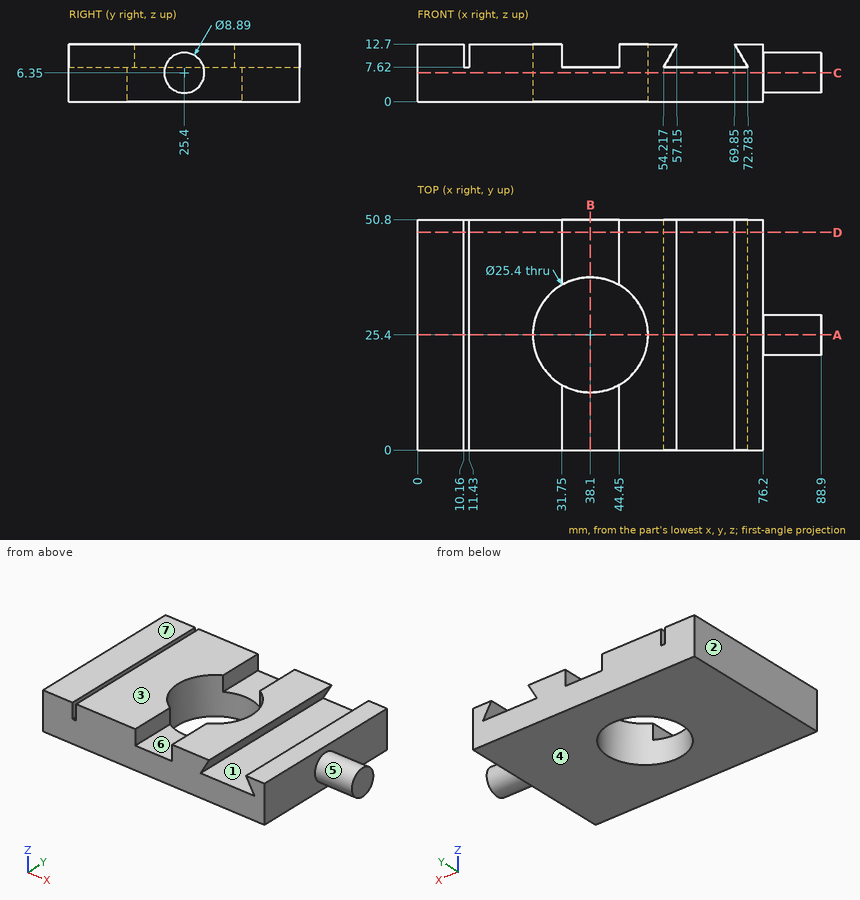
For this review, use the dimensioned drawing (mm, ordinates from the lowest corner) and the shaded views. A direction names the side the tool comes from. Give positions to 0.01 mm unless a question says otherwise; leave off trailing zeros. Order: outer loops, then holes, each group sorted by start corner. A loop starts at its lowest first (then second) coordinate and runs counter-clockwise, first axis right, second up. Notation, with made-up numbers: (-1, -32) - (43, -32) arc R21 cw to (43, -10) - close; hole circle Ø11 at (75, 85). An arc over 180 degrees is marked (long way). Write item = value, one per line. Start each with the question number.
Q1. Clearance check with flat-ended pins moving along their axes: pin 1 Ø5.5 at (y, z) = (40.5, 9) entering from +X; pin 2 Ø5.5 at (x, y) = (66, 15) entering from +Z; pin 3 Ø15 at (x, y) = (38.1, 25.4) entering from +Z. State where each tip first meets the part, or that it passes through.
Q2. Mouldability with a two-part tool opening along Z and no side actions: class the marked faces 1, 2, 3 and 4 as released by +Z, released by -Z, zero draft, split by the parting line, or undercut.
Q3. We need section A-A on y = 25.4. State the section outline as (x, z) points (3 decimals), plus the area to 3 significant figures.
Q4. To check wall thickness, follow L1, parallel to X at y = 30, z = 12; L2, parallel to X at y = 25.4, z = 5.25; L3, parallel to X at y = 25.4, z = 10. State the ranges of each line that lie inside material, in increasing order. Write a range as from..to.
Q5. Tool access review of the marked faces 5, 6 and 7: name each direction out of +Z, -Z, +X, -X, +Y, -Y from which nothing blocks a thin tool from reaching the whole face with its end or side.
Q6. We need section B-B on x = 38.1. State the section outline as (y, z) points.
Q7. We need section D-D on y = 48. State the section outline as (x, z) points.
Q8. We need section C-C on z = 6.35. State the section outline as (x, y) points (3 decimals), plus the area to 3 significant figures.
Working result:
q1.pin_1 = 76.2
q1.pin_2 = 7.62
q1.pin_3 = through
q2.face_1 = undercut
q2.face_2 = zero draft
q2.face_3 = released by +Z
q2.face_4 = released by -Z
q3.outline = (0, 0) - (25.4, 0) - (25.4, 12.7) - (11.43, 12.7) - (11.43, 7.62) - (10.16, 7.62) - (10.16, 12.7) - (0, 12.7) - close; (50.8, 0) - (76.2, 0) - (76.2, 1.905) - (88.9, 1.905) - (88.9, 10.795) - (76.2, 10.795) - (76.2, 12.7) - (69.85, 12.7) - (72.783, 7.62) - (54.217, 7.62) - (57.15, 12.7) - (50.8, 12.7) - close
q3.area = 672 mm²
q4.L1 = 0..10.16, 11.43..26.26, 49.94..56.75, 70.25..76.2
q4.L2 = 0..25.4, 50.8..88.9
q4.L3 = 0..10.16, 11.43..25.4, 50.8..55.59, 71.41..88.9
q5.face_5 = +X
q5.face_6 = +Z, +Y, -Y
q5.face_7 = +Z, +X, -X, +Y, -Y
q6.outline = (0, 0) - (12.7, 0) - (12.7, 7.62) - (0, 7.62) - close; (38.1, 0) - (50.8, 0) - (50.8, 7.62) - (38.1, 7.62) - close
q7.outline = (0, 0) - (76.2, 0) - (76.2, 12.7) - (69.85, 12.7) - (72.78, 7.62) - (54.22, 7.62) - (57.15, 12.7) - (44.45, 12.7) - (44.45, 7.62) - (31.75, 7.62) - (31.75, 12.7) - (11.43, 12.7) - (11.43, 7.62) - (10.16, 7.62) - (10.16, 12.7) - (0, 12.7) - close
q8.outline = (0, 0) - (76.2, 0) - (76.2, 20.955) - (88.9, 20.955) - (88.9, 29.845) - (76.2, 29.845) - (76.2, 50.8) - (0, 50.8) - close; hole circle Ø25.4 at (38.1, 25.4)
q8.area = 3,480 mm²
